Verification items for the finished model (mm, model axes). A direction names the side the tool comes from. Round coordinates to 2 decimals unless told otherwise and drop trailing zeros. Loops run counter-clockwise (first coordinate to the right, second up) from the corner with the lowest first, then second, coordinate; pieces in that order, holes last. Notation, with made-up numbers: (-13, 48.5) - (41, 48.5) arc R18 cw to (41, 71.5) - close; hole circle Ø5 at (19, 48.25). An arc over 180 degrees is marked (long way). Use CSV: the item, a comma, the result in double quotes.
```python
from build123d import *

# Parameters (mm, degrees)
F1_DEPTH = 3.8
F3_DEPTH = 4.5


with BuildPart() as f1:
    # F0 (on Top) → F1 (new body)
    with BuildSketch(Plane.XY):
        with BuildLine():
            Line((4.5, -7.6), (4.5, 0))
            Line((4.5, 0), (0, 0))
            Line((0, 0), (0, -5.3))
            ThreePointArc((0, -5.3), (1.202082, -5.797918), (1.7, -7))
            Line((1.7, -7), (1.7, -9.6))
            Line((1.7, -9.6), (2.5, -9.6))
            ThreePointArc((2.5, -9.6), (3.914214, -9.014214), (4.5, -7.6))
        make_face()
    extrude(amount=F1_DEPTH)

    # F2 (on face) → F3 (join, through all)
    with BuildSketch(Plane.YZ.offset(4.5)):
        Polygon((-3.6, 4.5), (-3.6, 3.8), (0, 3.8), (0, 5.5), (-2.6, 5.5), align=None)
    extrude(amount=-F3_DEPTH)

    # F4: F1 across face


with BuildPart() as f1_1:
    add(f1.part)
    add(f1.part.mirror(Plane(origin=(0, -2.43609, 2.489933), x_dir=(0, -1, 0), z_dir=(-1, 0, 0))))

    # F5: F1 across face


with BuildPart() as f1_2:
    add(f1_1.part)
    add(f1_1.part.mirror(Plane(origin=(0, 0, 2.75), x_dir=(-1, 0, 0), z_dir=(0, 1, 0))))


solid = f1_2.part
```
1) Mould release check, pull along X, two halves, no side actions. Record for faces 6 (the face through (0, 5, 3.8)), 7 (the face through (-3.9, -9.03, 1.87)), 8 (the face through (-1.7, -8, 2)): +X half, -X half, draft (parallel to the pull), parting line (faces both ways), or undercut.
Returned:
face 6,"draft"
face 7,"-X half"
face 8,"undercut"
2) Thickness scan on probe 1 along Z at (x, y) = (-1.75, -5.5); probe 2 along Y at (x, z) = (-0.5, 4.25); probe 3 along X at (y, z) = (6.5, 2.65). Record the ranges inside material, lowest first. Write a range as [from, to].
Returned:
probe 1,"z = [0, 3.8]"
probe 2,"y = [-3.6, 3.6]"
probe 3,"x = [-4.5, -1.62], [1.62, 4.5]"
3) Cross-section at B-B, the plane y = 8.25. Record the cut outline in (x, z), then the cut area to 3 significant figures.
Returned:
outline,"(-4.39, 0) - (-1.7, 0) - (-1.7, 3.8) - (-4.39, 3.8) - close; (1.7, 0) - (4.39, 0) - (4.39, 3.8) - (1.7, 3.8) - close"
area,"20.5 mm²"
4) Access from +Z, -Z, +X, -X, +Y, -Y to the whole of each face (thin tool, end or side, straight path). Record for faces 1 (the face through (3.9, -9.03, 1.87)), 2 (the face through (3.9, 9.03, 1.87)), 3 (the face through (0, -5, 3.8)), 4 (the face through (1.7, -8, 2)), 5 (the face through (-1.7, 8, 2)).
Returned:
face 1,"+Z, -Z, +X, -Y"
face 2,"+Z, -Z, +X, +Y"
face 3,"+Z, +X, -X, -Y"
face 4,"+Z, -Z, -Y"
face 5,"+Z, -Z, +Y"
5) Cross-section at C-C, the plane z = 0.6. Record the cut outline in (x, y), then the cut area to 3 significant figures.
Returned:
outline,"(-4.5, -7.6) arc R2 ccw to (-2.5, -9.6) - (-1.7, -9.6) - (-1.7, -7) arc R1.7 cw to (0, -5.3) arc R1.7 cw to (1.7, -7) - (1.7, -9.6) - (2.5, -9.6) arc R2 ccw to (4.5, -7.6) - (4.5, 7.6) arc R2 ccw to (2.5, 9.6) - (1.7, 9.6) - (1.7, 7) arc R1.7 cw to (0, 5.3) arc R1.7 cw to (-1.7, 7) - (-1.7, 9.6) - (-2.5, 9.6) arc R2 ccw to (-4.5, 7.6) - close"
area,"143 mm²"
6) Cross-section at A-A, the plane x = -2. Record the cut outline in (y, z), then the cut area to 3 significant figures.
Returned:
outline,"(-9.6, 0) - (9.6, 0) - (9.6, 3.8) - (3.6, 3.8) - (3.6, 4.5) - (2.6, 5.5) - (-2.6, 5.5) - (-3.6, 4.5) - (-3.6, 3.8) - (-9.6, 3.8) - close"
area,"84.2 mm²"
7) Cross-section at D-D, the plane x = 1.5. Record the cut outline in (y, z), then the cut area to 3 significant figures.
Returned:
outline,"(-6.2, 0) - (6.2, 0) - (6.2, 3.8) - (3.6, 3.8) - (3.6, 4.5) - (2.6, 5.5) - (-2.6, 5.5) - (-3.6, 4.5) - (-3.6, 3.8) - (-6.2, 3.8) - close"
area,"58.4 mm²"
8) Gauge pin test, flat ends, axial feed: pin 1 Ø0.8 at (y, z) = (-8.5, 1.5) entering from +X; pin 2 Ø3 at (x, y) = (1.5, 6.5) entering from +Z; pin 3 Ø1 at (x, z) = (-1, 2) entering from +Y. Record the tip position at first contact, or that the pin passes through.
Returned:
pin 1,"stops at x = 4.44"
pin 2,"stops at z = 3.8"
pin 3,"stops at y = 6.2"
